```python
from build123d import *

# Parameters (mm, degrees)
SKETCH1_R               = 3
BOSS_EXTRUDE1_DEPTH     = 20
SKETCH1_3_R             = 8.5
SKETCH1_3_R_2           = 3
BOSS_EXTRUDE2_DEPTH     = 10
SKETCH2_W               = 15
SKETCH2_H               = 6
CUT_EXTRUDE1_DEPTH      = 0.5
CUT_EXTRUDE1_DEPTH_BACK = 0.5


with BuildPart() as part:
    # Sketch1 → Boss-Extrude1 (new body)
    with BuildSketch(Plane.XY):
        Circle(SKETCH1_R)
    extrude(amount=BOSS_EXTRUDE1_DEPTH)

    # Sketch1_3 → Boss-Extrude2 (add)
    with BuildSketch(Plane.XY):
        Circle(SKETCH1_3_R)
        Circle(SKETCH1_3_R_2, mode=Mode.SUBTRACT)
        Circle(SKETCH1_3_R_2)
    extrude(amount=-BOSS_EXTRUDE2_DEPTH)

    # Sketch2 → Cut-Extrude1 (cut, two sides)
    with BuildSketch(Plane(origin=(0, 0, 0), x_dir=(0, 0, -1), z_dir=(1, 0, 0))) as cut_extrude1_sk:
        with Locations((-12.5, 0)):
            Rectangle(SKETCH2_W, SKETCH2_H)
    extrude(amount=CUT_EXTRUDE1_DEPTH, mode=Mode.SUBTRACT)
    extrude(cut_extrude1_sk.sketch, amount=-CUT_EXTRUDE1_DEPTH_BACK, mode=Mode.SUBTRACT)


solid = part.part
```
Work out the finished part from the listing and answer in its coordinate system (mm). A direction names the side the tool comes from. Coordinates: 2 decimals unless noted, no trailing zeros. Loops run counter-clockwise (first coordinate to the right, second up) from the corner with the lowest first, then second, coordinate; pieces in that order, holes last.
1) Section D-D (z = -5.75) is taken. Give the vertices of the cut face in (x, y), plus the area to 3 significant figures.
Results:
outline: circle Ø17 at (0, 0)
area: 227 mm2
2) For a pull along X with two mould halves and no side action, classify faces 1 (the cylindrical face through (-0.65, -2.93, 9.86)), 2 (the flat face through (1, 0, 20)), 3 (the flat face through (0.5, 0, 13)) as +X half, -X half, draft (parallel to the pull), parting line (faces both ways), or undercut.
Results:
face 1: parting line
face 2: draft
face 3: undercut
3) Flat-ended cylindrical pins translate along their axes: pin 1 (8 mm diameter, centred on x = -4, y = 6, fed in from +Z); pin 2 (6.5 mm diameter, centred on y = -1, z = 9.5, fed in from -X); pin 3 (10 mm diameter, centred on x = -5, z = 3, fed in from -Y); pin 4 (4 mm diameter, centred on y = 6, z = 10.5, fed in from +X). Find the tip coordinate at first contact, or state that the pin passes through.
Results:
pin 1: stops at z = 0
pin 2: stops at x = -3
pin 3: stops at y = -8.44
pin 4: passes through
4) For faces 4 (the flat face through (4, 0, 0)), 5 (the flat face through (-1, 0, 20)), 6 (the flat face through (-0.5, 0, 13)), determine the directions among +Z, -Z, +X, -X, +Y, -Y from which every point of the face is accessible in a straight line to the end or side of a thin tool.
Results:
face 4: +Z
face 5: +Z, +X, -X, +Y, -Y
face 6: +Z, +Y, -Y
5) Consider probe 1 along Z at (x, y) = (3, 3); probe 2 along X at (y, z) = (-1.25, 15.5); probe 3 along Y at (x, z) = (-0.25, -4). Determine where each line is inside the solid, lowest interval first.
Results:
probe 1: z = -10 to 0
probe 2: x = -2.73 to -0.5, 0.5 to 2.73
probe 3: y = -8.5 to 8.5
6) Section C-C (z = 9.5) is taken. Give the vertices of the cut face in (x, y), plus the area to 3 significant figures.
Results:
outline: (-0.5, -2.96) - (-0.5, 2.96) arc R3 ccw to start; (0.5, -2.96) arc R3 ccw to (0.5, 2.96) - close
area: 22.3 mm2
7) Section A-A (y = 0) is taken. Give the vertices of the cut face in (x, z).
Results:
outline: (-8.5, -10) - (8.5, -10) - (8.5, 0) - (3, 0) - (3, 20) - (0.5, 20) - (0.5, 5) - (-0.5, 5) - (-0.5, 20) - (-3, 20) - (-3, 0) - (-8.5, 0) - close
8) Section B-B (x = 0) is taken. Give the vertices of the cut face in (y, z), plus the area to 3 significant figures.
Results:
outline: (-8.5, -10) - (8.5, -10) - (8.5, 0) - (3, 0) - (3, 5) - (-3, 5) - (-3, 0) - (-8.5, 0) - close
area: 200 mm2
